from build123d import *

# Parameters (mm, degrees)
F0_W         = 30.48
F0_H         = 20.32
F1_DEPTH     = 2.54
F2_R         = 3.6195
F4_DEPTH     = 25.4
F5_DEPTH     = 1.524
F6_DEPTH     = 21.59
F7_W         = 27.94
F7_H         = 15.24
F8_DEPTH     = 15.621
F10_DEPTH    = 25.4
F11_W        = 2.54
F11_H        = 15.24
F12_DEPTH    = 4.572
F13_W        = 2.54
F13_H        = 15.24
F14_DEPTH    = 2.54
F15_R        = 9.9953269909
F16_T1_DEPTH = 15.24


# Not quite as in the source:
# - a fillet or chamfer that OpenCascade refuses, or shapes differently, is made with other operations: its cross-section is extruded or revolved along the edge and cut away or added


with BuildPart() as f1:
    # F0 (on Front) → F1 (new body)
    with BuildSketch(Plane.XZ):
        Rectangle(F0_W, F0_H)
    extrude(amount=F1_DEPTH)

    # F2 (on face) → F4 (cut)
    with BuildSketch(Plane.XZ.offset(2.54)):
        with Locations((-7.62, 0)):
            Circle(F2_R)
    extrude(amount=-F4_DEPTH, mode=Mode.SUBTRACT)

    # F3 (on face) → F5 (cut)
    with BuildSketch(Plane.XZ.offset(2.54)):
        Polygon((7.1528805111, 2.0839335623), (-6.0890655676, 3.2650576724), (-5.9136119671, -3.1920422334), (7.1528805111, -2.0996773468), (8.7022805111, -1.0994056345), (8.7022805111, 1.1413069921), align=None)
    extrude(amount=-F5_DEPTH, mode=Mode.SUBTRACT)

    # F6 (add): a face of the model
    f6_faces = [f1.faces().sort_by_distance(p)[0] for p in [
        (15.24, -1.27, 0),
    ]]
    extrude(f6_faces, amount=F6_DEPTH)

    # F7 (on face) → F8 (join)
    with BuildSketch(Plane.XZ.offset(2.54)):
        with Locations((22.86, 0)):
            Rectangle(F7_W, F7_H)
    extrude(amount=F8_DEPTH)

    # F9 (on face) → F10 (cut)
    with BuildSketch(Plane.XZ.offset(18.161)):
        Polygon((10.16, 6.35), (10.16, -6.35), (35.56, -6.35), (35.56, 0), (35.56, 6.35), align=None)
    extrude(amount=-F10_DEPTH, mode=Mode.SUBTRACT)

    # F11 (on face) → F12 (join)
    with BuildSketch(Plane(origin=(8.89, 0, 0), x_dir=(0, -1, 0), z_dir=(-1, 0, 0))):
        with Locations((16.891, 0)):
            Rectangle(F11_W, F11_H)
    extrude(amount=F12_DEPTH)

    # F13 (on face) → F14 (join, symmetric)
    with BuildSketch(Plane.YZ.offset(36.83)):
        with Locations((-16.891, 0)):
            Rectangle(F13_W, F13_H)
    extrude(amount=F14_DEPTH, both=True)

    # F15
    f15_edges = [f1.edges().sort_by_distance(p)[0] for p in [
        (-15.24, -1.27, 10.16),
        (-15.24, -1.27, -10.16),
    ]]
    fillet(f15_edges, radius=F15_R)

    # F16: fillet of radius 6.1321024484 on 2 edges, made by hand

    # F16_s2 → F16_t1 (join)
    with BuildSketch(Plane.XY.offset(-7.62)):
        with BuildLine():
            ThreePointArc((8.89, -9.6906744787), (7.6143050963, -13.4347346007), (4.318, -15.621))
            Line((4.318, -15.621), (8.89, -15.621))
            Line((8.89, -15.621), (8.89, -9.6906744787))
        make_face()
        with BuildLine():
            ThreePointArc((36.83, -10.6511428151), (37.5017993132, -13.4418004633), (39.37, -15.621))
            Line((39.37, -15.621), (36.83, -15.621))
            Line((36.83, -15.621), (36.83, -10.6511428151))
        make_face()
    extrude(amount=F16_T1_DEPTH)


solid = f1.part
CAD build for the part. Positions are in the model's coordinates, mm. A direction names the side the tool comes from. Round coordinates to 2 decimals unless told otherwise and drop trailing zeros. Write each loop counter-clockwise with the first axis right and the second up, starting at its lowest first coordinate (ties: lowest second). Pieces come first, ordered by that corner, then holes. Notation, with made-up numbers: M 18,2.25 L 56,2.25 A17 cw 56,15.25 Z; hole C 70,5 d8. An arc over 180 degrees is marked long. Put each result on its own line as item: value. Start each with the question number.
1) Drill centre lines: probe 1 along X at (y, z) = (-1.7, 0); probe 2 along Z at (x, y) = (23, -10.75); probe 3 along X at (y, z) = (-5, 5.5). Where is each one in solid material? Low to high. Write a range as [from, to].
2) Saw through at B-B, the plane y = -5. Write the cut outline in (x, z).
3) Pin check, flat tips, straight feed: pin 1 Ø5 at (y, z) = (-7.5, -7) entering from +X; pin 2 Ø10 at (y, z) = (-11, -0.5) entering from -X; pin 3 Ø4 at (y, z) = (-4, -5) entering from -X; pin 4 Ø12 at (x, z) = (30, -1) entering from +Y. Stop position of each tip, or through.
4) 3-axis set-ups, long thin cutter, end or side, ignore diameter. For faces 4 (the flat face through (22, -10, -7.62)), 5 (the flat face through (35.56, -8, 0)), 6 (the flat face through (22, -10, 7.62)), 7 (the flat face through (7.938, -1.789, 1.606)), 8 (the flat face through (10.16, -9, 0)): which of +Z, -Z, +X, -X, +Y, -Y reach the whole face in a straight line?
5) Saw through at A-A, the plane x = 15. Write the cut outline in (y, z).
6) Saw through at D-D, the plane y = -14. Write the cut outline in (x, z), and give its area (3 significant figures).
7) Saw through at C-C, the plane x = -7.62. Write the cut outline in (y, z).
8) Pull direction X, two halves, no side cores. Call faces 1 (the cylindrical face through (37.483, -13.406, -0.107)), 2 (the flat face through (23, -9, -6.35)), 3 (the flat face through (15, -1, -10.16)): pulls with the +X half, pulls with the -X half, needs draft (parallel to the pull), parting line crosses it, or undercut.
Resolved:
1. probe 1: [-15.24, -11.24], [8.7, 10.16], [35.56, 36.83]
1. probe 2: [-7.62, -6.35], [6.35, 7.62]
1. probe 3: [8.89, 10.16], [35.56, 36.83]
2. outline: M 8.89,-7.62 L 36.83,-7.62 L 36.83,7.62 L 8.89,7.62 Z; hole M 10.16,-6.35 L 35.56,-6.35 L 35.56,6.35 L 10.16,6.35 Z
3. pin 1: x = 36.83
3. pin 2: x = 4.32
3. pin 3: x = -14.62
3. pin 4: y = 0
4. face 4: -Z, +X, -X, -Y
4. face 5: +Y
4. face 6: +Z, +X, -X, -Y
4. face 7: none
4. face 8: +Y, -Y
5. outline: M -18.16,-7.62 L -2.54,-7.62 L -2.54,-10.16 L 0,-10.16 L 0,-6.35 L -18.16,-6.35 Z; M -18.16,6.35 L 0,6.35 L 0,10.16 L -2.54,10.16 L -2.54,7.62 L -18.16,7.62 Z
6. outline: M 7.12,-7.62 L 37.83,-7.62 L 37.83,7.62 L 7.12,7.62 Z; hole M 10.16,-6.35 L 35.56,-6.35 L 35.56,6.35 L 10.16,6.35 Z
6. area: 145 mm²
7. outline: M -2.54,-9.87 L 0,-9.87 L 0,-3.62 L -2.54,-3.62 Z; M -2.54,3.62 L 0,3.62 L 0,9.87 L -2.54,9.87 Z
8. face 1: pulls with the +X half
8. face 2: undercut
8. face 3: needs draft
